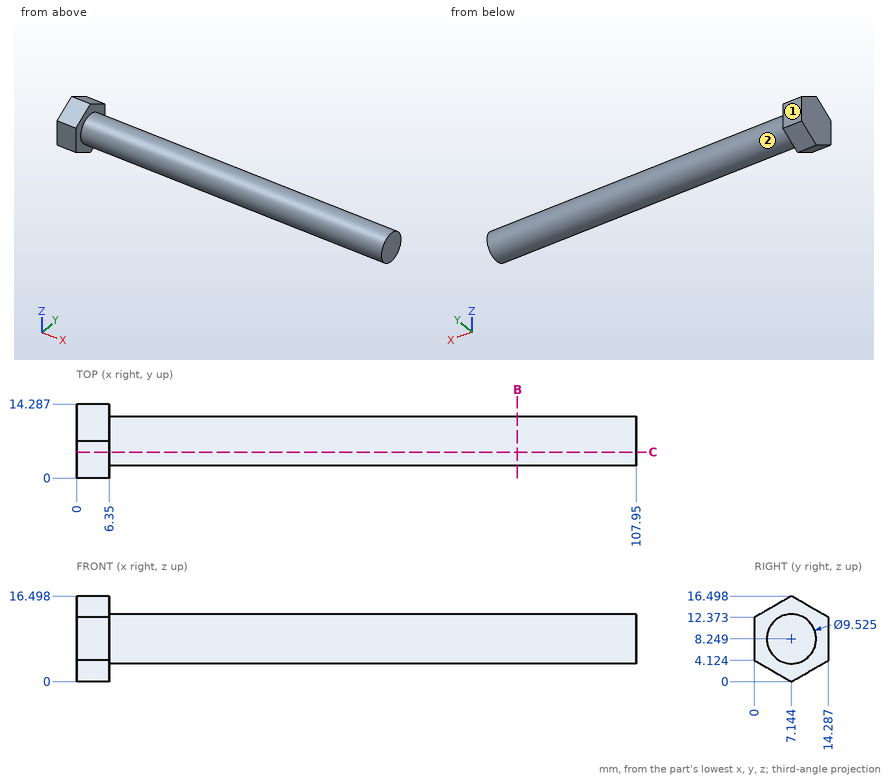
Part print with two shaded views. Sizes in mm from the minimum x, y, z corner. A direction names the side the tool comes from. Round coordinates to 2 decimals unless told otherwise and drop trailing zeros. Order: outer loops, then holes, each group sorted by start corner. A loop starts at its lowest first (then second) coordinate and runs counter-clockwise, first axis right, second up. Notation, with made-up numbers: M 56,70 L 62,70 A22 ccw 62,107 Z; hole C 66,-30 d10. An arc over 180 degrees is marked long. Answer in a Markdown table with one row per item. Add a question column.
Q1. Wall check: L1, parallel to X at y = 9.75, z = 14.5; L2, parallel to Z at x = 31, y = 7.25; L3, parallel to Y at x = 24.5, z = 8.25. Give the ranges that are in metal, low to high. Write a range as from..to.
Q2. Cut at C-C on y = 5. Give the cut face in (x, z).
Q3. 3-axis set-ups, long thin cutter, end or side, ignore diameter. For the marked faces 1 and 2: which of +Z, -Z, +X, -X, +Y, -Y reach the whole face in a straight line?
Q4. Pin check, flat tips, straight feed: pin 1 (5 mm diameter, centred on x = 65.5, z = 14.5, fed in from -Y); pin 2 (1.5 mm diameter, centred on x = 34.5, y = 3, fed in from -Z); pin 3 (8 mm diameter, centred on x = 43, y = 8.5, fed in from +Z). Stop position of each tip, or through.
Q5. Cut at B-B on x = 85. Give the cut face in (y, z) (1 decimal).
Established:
| question | item | result |
|---|---|---|
| 1 | L1 | x = 0..6.35 |
| 1 | L2 | z = 3.49..13.01 |
| 1 | L3 | y = 2.38..11.91 |
| 2 | outline | M 0,1.24 L 6.35,1.24 L 6.35,4 L 107.95,4 L 107.95,12.5 L 6.35,12.5 L 6.35,15.26 L 0,15.26 Z |
| 3 | face 1 | +Z, -Z, +X, -X, +Y |
| 3 | face 2 | +X |
| 4 | pin 1 | stops at y = 4.21 |
| 4 | pin 2 | stops at z = 4.91 |
| 4 | pin 3 | stops at z = 13.01 |
| 5 | outline | C 7.1,8.2 d9.5 |
